Design review of the part shown in the three views and the two pictorial views. Dimensions are in mm from the part's minimum x, y and z. Round coordinates to 2 decimals unless told otherwise and drop trailing zeros. Order: outer loops, then holes, each group sorted by start corner. A loop starts at its lowest first (then second) coordinate and runs counter-clockwise, first axis right, second up.
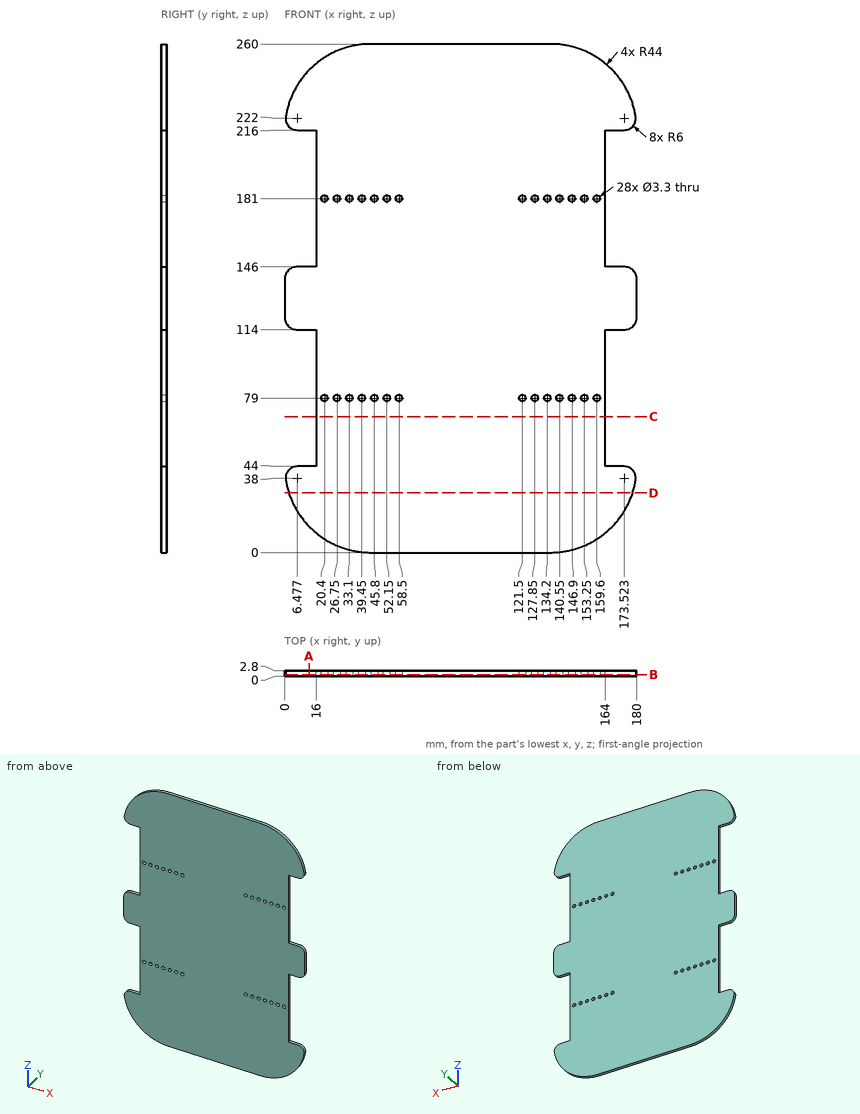
(1) Consider section A-A (x = 12.5). Write out the cut boundary in (y, z), and give its area (3 significant figures).
Data:
outline: (0, 13.28) - (2.8, 13.28) - (2.8, 44) - (0, 44) - close; (0, 114) - (2.8, 114) - (2.8, 146) - (0, 146) - close; (0, 216) - (2.8, 216) - (2.8, 246.72) - (0, 246.72) - close
area: 262 mm2
(2) To check wall thickness, follow probe 1 along Z at (x, y) = (45.8, 1.85); probe 2 along X at (y, z) = (2.5, 221.5); probe 3 along Z at (x, y) = (153.25, 0.65). State the ranges of each line that lie inside material, in increasing order.
Data:
probe 1: z = 0 to 77.35, 80.65 to 179.35, 182.65 to 260
probe 2: x = 0.5 to 179.5
probe 3: z = 3.52 to 77.35, 80.65 to 179.35, 182.65 to 256.48
(3) Consider section D-D (z = 30.5). Write out the cut boundary in (x, y).
Data:
outline: (2.12, 0) - (177.88, 0) - (177.88, 2.8) - (2.12, 2.8) - close
(4) Consider section B-B (y = 0.75). State how many separate pieces and enclosed holes the cut face has, and give its area (3 significant figures).
Data:
separate pieces: 1
enclosed holes: 28
area: 40,300 mm2
(5) Consider section C-C (z = 69.5). Write out the cut boundary in (x, y).
Data:
outline: (16, 0) - (164, 0) - (164, 2.8) - (16, 2.8) - close
(6) Insertion check: pin 1 (0.8 mm diameter, centred on x = 171, y = 1.5, fed in from +Z); pin 2 (2 mm diameter, centred on x = 153.25, z = 181, fed in from -Y); pin 3 (4.5 mm diameter, centred on x = 58.5, z = 79, fed in from +Y); pin 4 (1 mm diameter, centred on y = 2, z = 67, fed in from -X). Each pin has a flat end and moves straight along its axis. Give the tip position at first contact, or say it passes through.
Data:
pin 1: stops at z = 243.18
pin 2: passes through
pin 3: stops at y = 2.8
pin 4: stops at x = 16
